The figure shows three views and two pictorial views of one solid part (mm, origin at its lowest corner). Answer the questions. Round coordinates to 2 decimals unless told otherwise and drop trailing zeros. Order: outer loops, then holes, each group sorted by start corner. A loop starts at its lowest first (then second) coordinate and runs counter-clockwise, first axis right, second up. Notation, with made-up numbers: (50.5, -27.5) - (72.5, -27.5) arc R17 cw to (72.5, 1.5) - close; hole circle Ø9 at (26.5, 73.5). An arc over 180 degrees is marked (long way). Use CSV: the item, a comma, the result in double quotes.
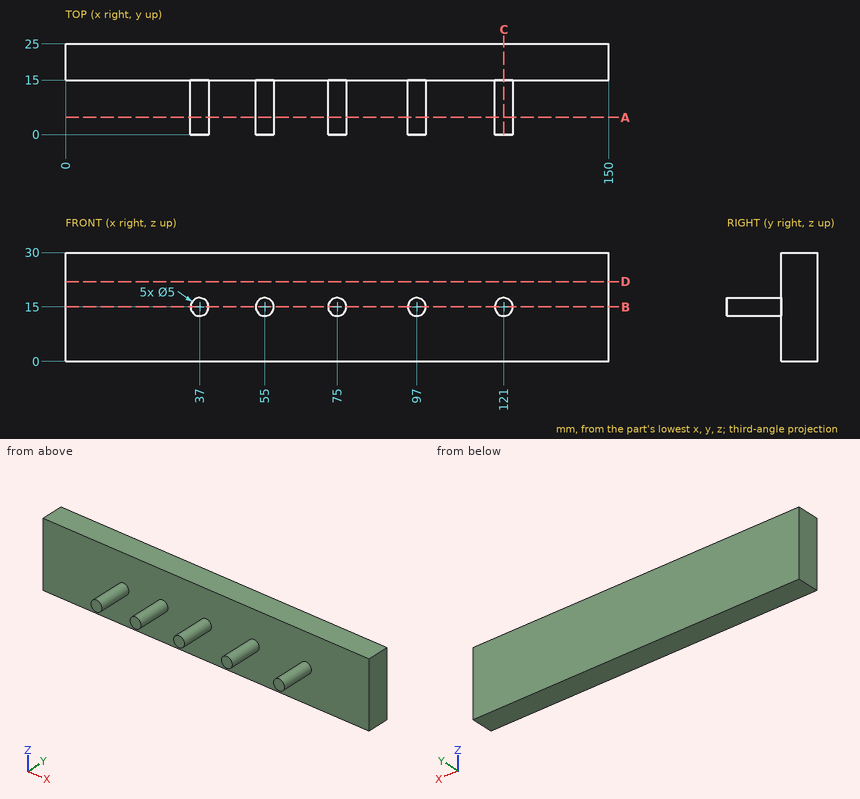
(1) Find section A-A (y = 4.75). Determine the outline of the cut face in (x, z), and give its area (3 significant figures).
Findings below:
outline,"circle Ø5 at (37, 15); circle Ø5 at (55, 15); circle Ø5 at (75, 15); circle Ø5 at (97, 15); circle Ø5 at (121, 15)"
area,"98.2 mm²"
(2) Find section D-D (z = 22). Determine the outline of the cut face in (x, y).
Findings below:
outline,"(0, 15) - (150, 15) - (150, 25) - (0, 25) - close"
(3) Find section C-C (x = 121). Determine the outline of the cut face in (y, z), and give its area (3 significant figures).
Findings below:
outline,"(0, 12.5) - (15, 12.5) - (15, 0) - (25, 0) - (25, 30) - (15, 30) - (15, 17.5) - (0, 17.5) - close"
area,"375 mm²"
(4) Find the intervals of material crossed by L1, parallel to X at y = 7, z = 15.25; L2, parallel to X at y = 13, z = 17; L3, parallel to Y at x = 65, z = 11.25, in increasing order. Write a range as from..to.
Findings below:
L1,"x = 34.51..39.49, 52.51..57.49, 72.51..77.49, 94.51..99.49, 118.51..123.49"
L2,"x = 35.5..38.5, 53.5..56.5, 73.5..76.5, 95.5..98.5, 119.5..122.5"
L3,"y = 15..25"
(5) Each of these flat-tipped pins is pushed along its axis until it touches: pin 1 (3 mm diameter, centred on x = 120.5, y = 6, fed in from -Z); pin 2 (4 mm diameter, centred on x = 124, z = 6.5, fed in from -Y); pin 3 (12 mm diameter, centred on x = 83, y = 6, fed in from +Z). Where does it stop, or does it pass through?
Findings below:
pin 1,"stops at z = 12.5"
pin 2,"stops at y = 15"
pin 3,"stops at z = 16.5"
(6) Find section B-B (z = 15). Determine the outline of the cut face in (x, y).
Findings below:
outline,"(0, 15) - (34.5, 15) - (34.5, 0) - (39.5, 0) - (39.5, 15) - (52.5, 15) - (52.5, 0) - (57.5, 0) - (57.5, 15) - (72.5, 15) - (72.5, 0) - (77.5, 0) - (77.5, 15) - (94.5, 15) - (94.5, 0) - (99.5, 0) - (99.5, 15) - (118.5, 15) - (118.5, 0) - (123.5, 0) - (123.5, 15) - (150, 15) - (150, 25) - (0, 25) - close"
